from build123d import *

# Parameters (mm, degrees)
F0_W     = 134.55
F0_H     = 82.69
F1_DEPTH = 13.01
F2_W     = 60.370001
F2_H     = 6.50506
F3_DEPTH = 82.691
F4_W     = 60.370001
F4_H     = 82.69
F5_DEPTH = 6.50494
F6_R     = 8.999995
F6_R_2   = 9.0043
F7_DEPTH = 13.011


with BuildPart() as f1:
    # F0 (on Top) → F1 (new body)
    with BuildSketch(Plane.XY):
        with Locations((-23.54345, -1.874108)):
            Rectangle(F0_W, F0_H)
    extrude(amount=F1_DEPTH)

    # F2 (on face) → F3 (cut, through all)
    with BuildSketch(Plane.XZ.offset(43.219108)):
        with Locations((-23.54345, 3.25253)):
            Rectangle(F2_W, F2_H)
    extrude(amount=-F3_DEPTH, mode=Mode.SUBTRACT)

    # F4 (on face) → F5 (join)
    with BuildSketch(Plane.XY.offset(13.01)):
        with Locations((-23.54345, -1.874108)):
            Rectangle(F4_W, F4_H)
    extrude(amount=F5_DEPTH)

    # F6 (on face) → F7 (cut, through all)
    with BuildSketch(Plane.XY.offset(13.01)):
        with Locations((27.131545, 22.870887)):
            Circle(F6_R)
        with Locations((27.127239, -26.614798)):
            Circle(F6_R_2)
        with Locations((-74.21414, 22.866582)):
            Circle(F6_R_2)
        with Locations((-74.21414, -26.614798)):
            Circle(F6_R_2)
    extrude(amount=-F7_DEPTH, mode=Mode.SUBTRACT)


solid = f1.part
Geometry: final body of the model. Coordinates: model frame, mm. A direction names the side the tool comes from. Give positions to 0.01 mm unless a question says otherwise; leave off trailing zeros. Loops run counter-clockwise (first coordinate to the right, second up) from the corner with the lowest first, then second, coordinate; pieces in that order, holes last. Notation, with made-up numbers: M 71,39 L 86,39 A15 ccw 86,66 Z; hole C -28,27 d9. An arc over 180 degrees is marked long. Put each result on its own line as item: value. Start each with the question number.
1) Cut plane C-C (x = -76). Output: boundary loops of the cut face in (y, z).
2) Cut plane A-A (z = 3.25). Output: boundary loops of the cut face in (x, y), then the cut area to 3 significant figures.
3) Pull-direction query (Y, two-part tool) for faces 4 (the flat face through (-24, -1, 19.515)), 5 (the flat face through (-24, 39.471, 10)), 6 (the cylindrical face through (20.49, -20.53, 6.6)), 7 (the cylindrical face through (35.445, 19.424, 6.596)); classes: pulls with the +Y half, pulls with the -Y half, needs draft (parallel to the pull), parting line crosses it, or undercut.
4) Contact query for flat-ended pins moving along their axis: pin 1 (11 mm diameter, centred on x = -74.21, y = -26.61, fed in from +Z); pin 2 (11 mm diameter, centred on x = -73.5, y = 13, fed in from +Z); pin 3 (1.5 mm diameter, centred on y = 27, z = 14, fed in from +X); pin 4 (18 mm diameter, centred on x = -27.5, y = 10, fed in from -Z). Output: stop coordinate, or through.
5) Access query for faces 1 (the flat face through (6.642, -2, 3)), 2 (the flat face through (25, -1, 13.01)), 3 (the flat face through (-73, -1, 13.01)). Directions: +Z, -Z, +X, -X, +Y, -Y. A direction counts if a zero-diameter tool reaches every point of the face in a straight line with its end or side. Return the directions, or none.
6) Cut plane B-B (y = 4.5). Output: boundary loops of the cut face in (x, z), then the cut area to 3 significant figures.
7) Ray query, line 1 along X through (y, z) = (1.5, 3); line 2 along X through (y, z) = (-33, 3.5); line 3 along X through (y, z) = (25, 8.75). Return the intervals inside material, ascending.
8) Cut plane D-D (z = 10.25). Output: boundary loops of the cut face in (x, y), then the cut area to 3 significant figures.
Verdict:
1. outline: M -43.22,0 L -35.44,0 L -35.44,13.01 L -43.22,13.01 Z; M -17.79,0 L 14.04,0 L 14.04,13.01 L -17.79,13.01 Z; M 31.69,0 L 39.47,0 L 39.47,13.01 L 31.69,13.01 Z
2. outline: M -90.82,-43.22 L -53.73,-43.22 L -53.73,39.47 L -90.82,39.47 Z; M 6.64,-43.22 L 43.73,-43.22 L 43.73,39.47 L 6.64,39.47 Z; hole C -74.21,-26.61 d18.01; hole C -74.21,22.87 d18.01; hole C 27.13,-26.61 d18.01; hole C 27.13,22.87 d18
2. area: 5,120 mm2
3. face 4: needs draft
3. face 5: pulls with the +Y half
3. face 6: undercut
3. face 7: undercut
4. pin 1: through
4. pin 2: z = 13.01
4. pin 3: x = 6.64
4. pin 4: z = 6.51
5. face 1: -Z, +Y, -Y
5. face 2: +Z, +X, +Y, -Y
5. face 3: +Z, -X, +Y, -Y
6. outline: M -90.82,0 L -53.73,0 L -53.73,6.51 L 6.64,6.51 L 6.64,0 L 43.73,0 L 43.73,13.01 L 6.64,13.01 L 6.64,19.51 L -53.73,19.51 L -53.73,13.01 L -90.82,13.01 Z
6. area: 1,750 mm2
7. line 1: -90.82 to -53.73, 6.64 to 43.73
7. line 2: -90.82 to -80.56, -67.87 to -53.73, 6.64 to 20.78, 33.48 to 43.73
7. line 3: -90.82 to -82.96, -65.47 to 18.39, 35.88 to 43.73
8. outline: M -90.82,-43.22 L 43.73,-43.22 L 43.73,39.47 L -90.82,39.47 Z; hole C -74.21,-26.61 d18.01; hole C -74.21,22.87 d18.01; hole C 27.13,-26.61 d18.01; hole C 27.13,22.87 d18
8. area: 10,100 mm2
